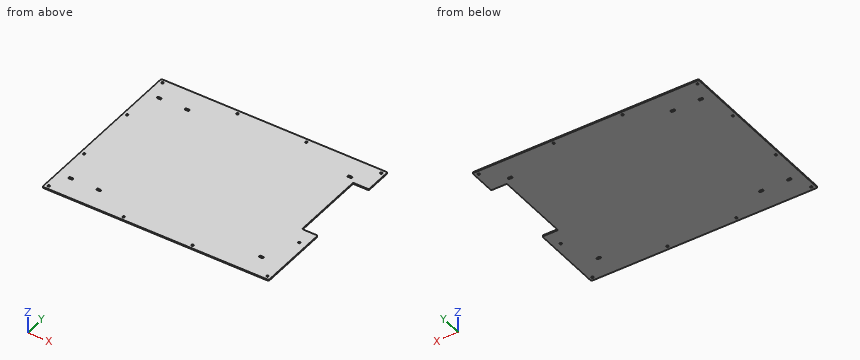
from build123d import *

# Parameters (mm, degrees)
SKETCH1_W                         = 604
SKETCH1_H                         = 470
BOSS_EXTRUDE1_DEPTH               = 3
FILLET1_R                         = 3
M5_CLEARANCE_HOLE1_D              = 5.5
M5_MANUFACTURING_FIXTURING_HOLE_D = 5.5
CUT_EXTRUDE5_DEPTH                = 766.326727614
SKETCH6_W                         = 42
SKETCH6_H                         = 202
CUT_EXTRUDE2_DEPTH                = 766.326727614
FILLET3_R                         = 3


with BuildPart() as part:
    # Sketch1 → Boss-Extrude1 (new body)
    with BuildSketch(Plane.XY):
        with Locations((302, 235)):
            Rectangle(SKETCH1_W, SKETCH1_H)
    extrude(amount=BOSS_EXTRUDE1_DEPTH)

    # Fillet1
    fillet1_edges = [part.edges().sort_by_distance(p)[0] for p in [
        (0, 470, 1.5),
        (604, 470, 1.5),
        (604, 0, 1.5),
        (0, 0, 1.5),
    ]]
    fillet(fillet1_edges, radius=FILLET1_R)

    # M5 Clearance Hole1 (through all)
    with Locations(Plane(origin=(0, 0, 0), x_dir=(-1, 0, 0), z_dir=(0, 0, -1))):
        with Locations((-594, 460), (-394, 460), (-210, 460), (-10, 460), (-10, 10), (-210, 10), (-394, 10), (-594, 10), (-544, 410), (-544, 60), (-35, 410), (-35, 60), (-109.625, 410), (-109.625, 60)):
            Hole(M5_CLEARANCE_HOLE1_D / 2)

    # M5 Manufacturing Fixturing Hole (through all)
    with Locations(Plane.XY.offset(3)):
        with Locations((10, 320), (10, 150), (584, 320), (584, 150)):
            Hole(M5_MANUFACTURING_FIXTURING_HOLE_D / 2)

    # Sketch9 → Cut-Extrude5 (cut, through all)
    with BuildSketch(Plane.XY.offset(3)):
        with BuildLine():
            Line((32, 412.75), (38, 412.75))
            ThreePointArc((38, 412.75), (40.75, 410), (38, 407.25))
            Line((38, 407.25), (32, 407.25))
            ThreePointArc((32, 407.25), (29.25, 410), (32, 412.75))
        make_face()
        with BuildLine():
            Line((106.625, 412.75), (112.625, 412.75))
            ThreePointArc((112.625, 412.75), (115.375, 410), (112.625, 407.25))
            Line((112.625, 407.25), (106.625, 407.25))
            ThreePointArc((106.625, 407.25), (103.875, 410), (106.625, 412.75))
        make_face()
        with BuildLine():
            Line((32, 62.75), (38, 62.75))
            ThreePointArc((38, 62.75), (40.75, 60), (38, 57.25))
            Line((38, 57.25), (32, 57.25))
            ThreePointArc((32, 57.25), (29.25, 60), (32, 62.75))
        make_face()
        with BuildLine():
            Line((106.625, 62.75), (112.625, 62.75))
            ThreePointArc((112.625, 62.75), (115.375, 60), (112.625, 57.25))
            Line((112.625, 57.25), (106.625, 57.25))
            ThreePointArc((106.625, 57.25), (103.875, 60), (106.625, 62.75))
        make_face()
        with BuildLine():
            Line((541, 412.75), (547, 412.75))
            ThreePointArc((547, 412.75), (549.75, 410), (547, 407.25))
            Line((547, 407.25), (541, 407.25))
            ThreePointArc((541, 407.25), (538.25, 410), (541, 412.75))
        make_face()
        with BuildLine():
            Line((541, 62.75), (547, 62.75))
            ThreePointArc((547, 62.75), (549.75, 60), (547, 57.25))
            Line((547, 57.25), (541, 57.25))
            ThreePointArc((541, 57.25), (538.25, 60), (541, 62.75))
        make_face()
    extrude(amount=-CUT_EXTRUDE5_DEPTH, mode=Mode.SUBTRACT)

    # Sketch6 → Cut-Extrude2 (cut, through all)
    with BuildSketch(Plane.XY.offset(3)):
        with Locations((583, 295)):
            Rectangle(SKETCH6_W, SKETCH6_H)
    extrude(amount=-CUT_EXTRUDE2_DEPTH, mode=Mode.SUBTRACT)

    # Fillet3
    fillet3_edges = [part.edges().sort_by_distance(p)[0] for p in [
        (604, 396, 1.5),
        (604, 194, 1.5),
        (562, 194, 1.5),
        (562, 396, 1.5),
    ]]
    fillet(fillet3_edges, radius=FILLET3_R)


solid = part.part
The listing builds one solid part. Answer for the finished solid, in the listing's coordinates (mm). Round coordinates to 2 decimals unless told otherwise and drop trailing zeros. Write each loop counter-clockwise with the first axis right and the second up, starting at its lowest first coordinate (ties: lowest second). Pieces come first, ordered by that corner, then holes. Notation, with made-up numbers: M 78.25,-13 L 107.25,-13 A11 ccw 107.25,-1 Z; hole C -6.75,78 d11. An arc over 180 degrees is marked long. Write each question's results on one line, items separated by ' | '. Start each with the question number.
(1) Find the intervals of material crossed by line 1 (Y direction, x = 10, z = 1.8); line 2 (X direction, y = 60.5, z = 1.15); line 3 (X direction, y = 460, z = 1.6), in increasing order.
(2) The part is cut by section A-A, the plane z = 0.9. Give the number of separate pieces and of enclosed holes in the cut face, and give its area (3 significant figures).
(3) The part is cut by section B-B, the plane y = 235. Write down the section's boundary in (x, z).
(4) Each of these flat-tipped pins is pushed along its axis until it touches: P1, Ø6.5, axis at x = 10, y = 320, coming from the +Z side; P2, Ø1.5, axis at y = 254.5, z = 1.5, coming from the +X side. Where does it stop, or does it pass through?
Worked answers:
1) line 1: y = 0 to 7.25, 12.75 to 147.25, 152.75 to 317.25, 322.75 to 457.25, 462.75 to 470 | line 2: x = 0 to 29.3, 40.7 to 103.92, 115.33 to 538.3, 549.7 to 604 | line 3: x = 0 to 7.25, 12.75 to 207.25, 212.75 to 391.25, 396.75 to 591.25, 596.75 to 604
2) separate pieces: 1 | enclosed holes: 17 | area: 275,000 mm²
3) outline: M 0,0 L 562,0 L 562,3 L 0,3 Z
4) P1: stops at z = 3 | P2: stops at x = 562
